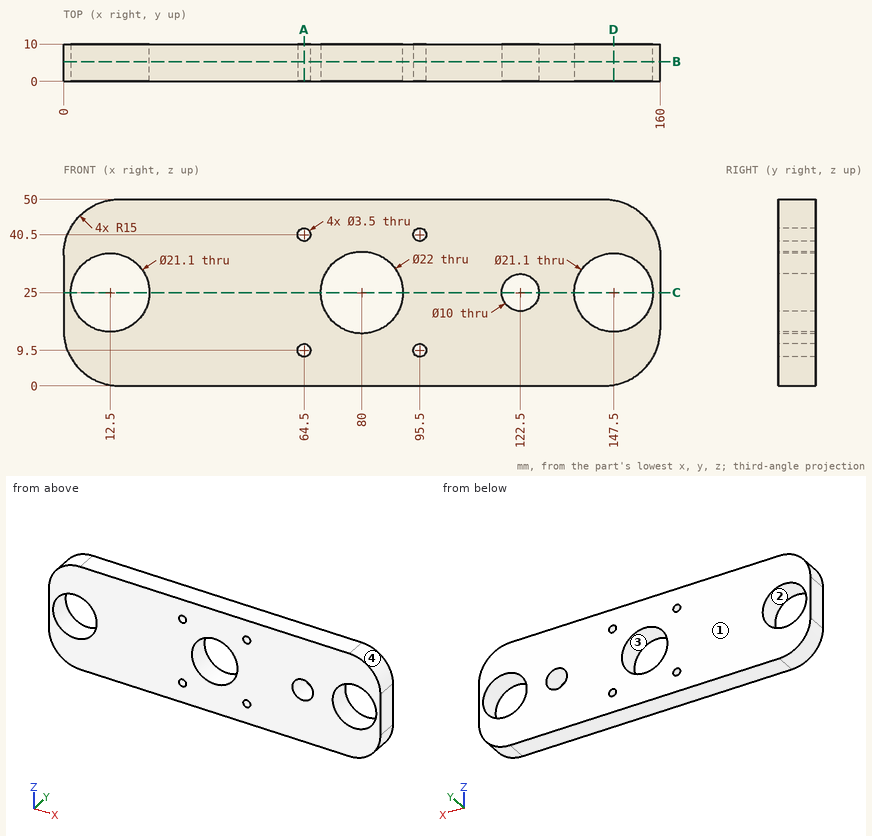
Print and shaded views of the part. All mm, measured from the part's lowest x, y and z. Give positions to 0.01 mm unless a question says otherwise; leave off trailing zeros. Loops run counter-clockwise (first coordinate to the right, second up) from the corner with the lowest first, then second, coordinate; pieces in that order, holes last. Notation, with made-up numbers: (-38.75, 84) - (-7.75, 84) arc R30 ccw to (-7.75, 114) - close; hole circle Ø5 at (81, 17). An arc over 180 degrees is marked (long way). Use a Markdown table: item, result.
(1) Band-saw the part on A-A (x = 64.5). Give the cut face in (y, z), and give its area (3 significant figures).
Taken from the geometry:
| item | result |
|---|---|
| outline | (0, 0) - (10, 0) - (10, 7.75) - (0, 7.75) - close; (0, 11.25) - (10, 11.25) - (10, 38.75) - (0, 38.75) - close; (0, 42.25) - (10, 42.25) - (10, 50) - (0, 50) - close |
| area | 430 mm2 |
(2) Band-saw the part on C-C (z = 25). Give the cut face in (x, y).
Taken from the geometry:
| item | result |
|---|---|
| outline | (0, 0) - (1.95, 0) - (1.95, 10) - (0, 10) - close; (23.05, 0) - (69, 0) - (69, 10) - (23.05, 10) - close; (91, 0) - (117.5, 0) - (117.5, 10) - (91, 10) - close; (127.5, 0) - (136.95, 0) - (136.95, 10) - (127.5, 10) - close; (158.05, 0) - (160, 0) - (160, 10) - (158.05, 10) - close |
(3) Wall check: line 1 along Z through (x, y) = (64.5, 6); line 2 along X through (y, z) = (8.25, 24.5); line 3 along X through (y, z) = (7.5, 21.5). Give the ranges that are in metal, low to high.
Taken from the geometry:
| item | result |
|---|---|
| line 1 | 0 to 7.75, 11.25 to 38.75, 42.25 to 50 |
| line 2 | 0 to 1.96, 23.04 to 69.01, 90.99 to 117.53, 127.47 to 136.96, 158.04 to 160 |
| line 3 | 0 to 2.55, 22.45 to 69.57, 90.43 to 118.93, 126.07 to 137.55, 157.45 to 160 |
(4) Pull direction X, two halves, no side cores. Call the marked faces 1, 2, 3 and 4: +X half, -X half, draft (parallel to the pull), parting line (faces both ways), or undercut.
Taken from the geometry:
| item | result |
|---|---|
| face 1 | draft |
| face 2 | undercut |
| face 3 | undercut |
| face 4 | +X half |
(5) Band-saw the part on B-B (y = 5.25). Give the number of separate pieces and of enclosed holes in the cut face, and give its area (3 significant figures).
Taken from the geometry:
| item | result |
|---|---|
| separate pieces | 1 |
| enclosed holes | 8 |
| area | 6,610 mm2 |
(6) Drop flat-ended pins along their axis: pin 1 Ø4 at (x, z) = (64.5, 40.5) entering from +Y; pin 2 Ø1.5 at (y, z) = (7.5, 36) entering from -X; pin 3 Ø19 at (x, z) = (12.5, 25) entering from +Y. Give the stop position or say it passes through.
Taken from the geometry:
| item | result |
|---|---|
| pin 1 | y = 10 |
| pin 2 | x = 0 |
| pin 3 | through |
(7) Band-saw the part on D-D (x = 147.5). Give the cut face in (y, z), and give its area (3 significant figures).
Taken from the geometry:
| item | result |
|---|---|
| outline | (0, 0.21) - (10, 0.21) - (10, 14.45) - (0, 14.45) - close; (0, 35.55) - (10, 35.55) - (10, 49.79) - (0, 49.79) - close |
| area | 285 mm2 |
